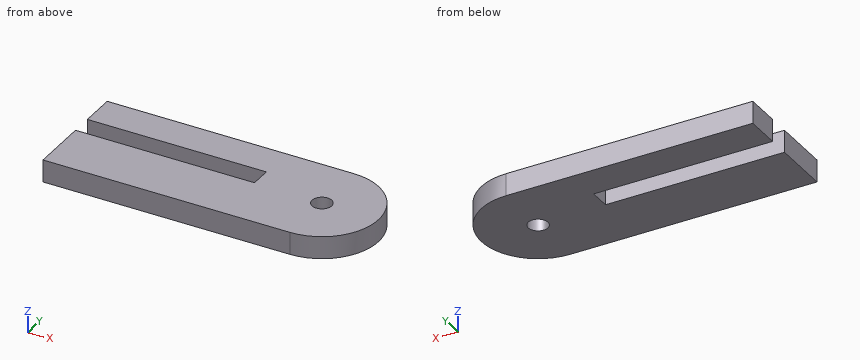
```python
from build123d import *

# Parameters (mm, degrees)
SKETCH1_R           = 1.3984
BOSS_EXTRUDE1_DEPTH = 3.175


with BuildPart() as part:
    # Sketch1 → Boss-Extrude1 (new body)
    with BuildSketch(Plane.XY):
        with BuildLine():
            Line((-0.1016, 15.9766), (34.925, 15.9766))
            ThreePointArc((34.925, 15.9766), (42.9641, 7.9375), (34.925, -0.1016))
            Line((34.925, -0.1016), (-0.1016, -0.1016))
            Line((-0.1016, -0.1016), (-0.1016, 4.7625))
            Line((-0.1016, 4.7625), (-0.1016, 8.0391))
            Line((-0.1016, 8.0391), (25.2984, 8.0391))
            Line((25.2984, 8.0391), (25.2984, 11.0109))
            Line((25.2984, 11.0109), (-0.1016, 11.0109))
            Line((-0.1016, 11.0109), (-0.1016, 15.9766))
        make_face()
        with Locations((34.925, 7.9375)):
            Circle(SKETCH1_R, mode=Mode.SUBTRACT)
    extrude(amount=BOSS_EXTRUDE1_DEPTH)


solid = part.part
```
The model under review builds one solid part; all positions refer to its coordinate system, in mm. Coordinates: 2 decimals unless noted, no trailing zeros. Write each loop counter-clockwise with the first axis right and the second up, starting at its lowest first coordinate (ties: lowest second). Pieces come first, ordered by that corner, then holes.
1) To check wall thickness, follow probe 1 along Y at (x, z) = (11.5, 0.85); probe 2 along X at (y, z) = (8, 1.8); probe 3 along Y at (x, z) = (35, 0.3). State the ranges of each line that lie inside material, in increasing order.
2) We need section C-C on y = 13.75. State the section outline as (x, z) points (3 decimals).
3) We need section D-D on x = 39.5. State the section outline as (y, z) points (3 decimals).
4) We need section B-B on z = 0.95. State the section outline as (x, y) points (1 decimal).
5) We need section A-A on x = 10.5. State the section outline as (y, z) points (3 decimals).
Answer list:
1. probe 1: y = -0.1 to 8.04, 11.01 to 15.98
1. probe 2: x = -0.1 to 33.53, 36.32 to 42.96
1. probe 3: y = -0.1 to 6.54, 9.33 to 15.98
2. outline: (-0.102, 0) - (40.479, 0) - (40.479, 3.175) - (-0.102, 3.175) - close
3. outline: (1.327, 0) - (14.548, 0) - (14.548, 3.175) - (1.327, 3.175) - close
4. outline: (-0.1, -0.1) - (34.9, -0.1) arc R8 ccw to (34.9, 16) - (-0.1, 16) - (-0.1, 11) - (25.3, 11) - (25.3, 8) - (-0.1, 8) - close; hole circle Ø2.8 at (34.9, 7.9)
5. outline: (-0.102, 0) - (8.039, 0) - (8.039, 3.175) - (-0.102, 3.175) - close; (11.011, 0) - (15.977, 0) - (15.977, 3.175) - (11.011, 3.175) - close
